Build history of the part. All positions in model axes, mm. Round coordinates to 2 decimals unless told otherwise and drop trailing zeros. Loops run counter-clockwise (first coordinate to the right, second up) from the corner with the lowest first, then second, coordinate; pieces in that order, holes last. Notation, with made-up numbers: (-27.75, 3.25) - (25.25, 3.25) arc R31 ccw to (25.25, 34.25) - close; hole circle Ø8 at (70, 5.25). An arc over 180 degrees is marked (long way). Use one line per item in the form item = value. Start each with the question number.
Q1. Mould opens along X. For faces 1 (the face through (-66, 1, 10)), 2 (the face through (0, -1, 10)), 3 (the face through (-37.893, 44.78, 10.14)), 4 (the face through (-50.856, -42.211, 10.14)) say: released by +X, released by -X, zero draft, split by the parting line, or undercut.
Q2. Saw through at B-B (z = 12.25). Give the cut face in (x, y), then the cut area to 3 significant figures.
Q3. Drill centre lines: line 1 (Y direction, x = -44, z = 14.25); line 2 (Y direction, x = -43, z = 15); line 3 (X direction, y = -37.5, z = 4.75). Where is each one in solid material? Low to high.
Q4. Pin check, flat tip, straight feed: pin 1 (13.5 mm diameter, centred on x = -43.84, y = 40.22, fed in from -Z). Stop position of the tip, or through.
Q5. Saw through at A-A (x = -46). Give the cut face in (y, z), then the cut area to 3 significant figures.
```python
from build123d import *

# Parameters (mm, degrees)
F0_W     = 22
F0_H     = 15
F0_W_2   = 44
F0_H_2   = 80
F1_DEPTH = 20
F3_D     = 15


with BuildPart() as f1:
    # F0 (on Top) → F1 (new body)
    with BuildSketch(Plane.XY):
        with Locations((-55, 47.5)):
            Rectangle(F0_W, F0_H)
        with Locations((-22, 47.5)):
            Rectangle(F0_W_2, F0_H)
        Polygon((0, -40), (0, 0), (0, 40), (-44, 40), (-44, -40), align=None)
        with Locations((-55, 0)):
            Rectangle(F0_W, F0_H_2)
        with Locations((-55, -47.5)):
            Rectangle(F0_W, F0_H)
        with Locations((-22, -47.5)):
            Rectangle(F0_W_2, F0_H)
    extrude(amount=F1_DEPTH)

    # F3 (through all)
    with Locations(Plane(origin=(0, 0, 0), x_dir=(1, 0, 0), z_dir=(0, 0, -1))):
        with Locations((-43.8447110355, -40.2159020305), (-43.7023043633, 39.95815292)):
            Hole(F3_D / 2)


solid = f1.part
```
Report:
q1.face_1 = released by -X
q1.face_2 = released by +X
q1.face_3 = undercut
q1.face_4 = undercut
q2.outline = (-66, -55) - (0, -55) - (0, 55) - (-66, 55) - close; hole circle Ø15 at (-43.84, 40.22); hole circle Ø15 at (-43.7, -39.96)
q2.area = 6,910 mm²
q3.line_1 = -55 to -47.45, -32.46 to 32.72, 47.71 to 55
q3.line_2 = -55 to -47.43, -32.49 to 32.76, 47.67 to 55
q3.line_3 = -66 to -50.79, -36.62 to 0
q4.pin_1 = through
q5.outline = (-55, 0) - (-47.1, 0) - (-47.1, 20) - (-55, 20) - close; (-32.82, 0) - (33.03, 0) - (33.03, 20) - (-32.82, 20) - close; (47.4, 0) - (55, 0) - (55, 20) - (47.4, 20) - close
q5.area = 1,630 mm²
